Autodesk Inventor part; units mm, degrees
ref_plane "YZ Plane" through (0, 0, 0) normal (1, 0, 0) x (0, 1, 0)
ref_plane "XZ Plane" through (0, 0, 0) normal (0, 1, 0) x (-1, 0, 0)
ref_plane "XY Plane" through (0, 0, 0) normal (0, 0, 1) x (1, 0, 0)
sketch "Boceto1" plane through (0, 0, 0) normal (0, 1, 0) x (-1, 0, 0)
  circle A0 centre (0, 0) radius 7.95
  dimension "d0" = 15.9
extrude "Extrusión1" add sketch "Boceto1" along normal blind 1.3
sketch "Boceto2" plane through (0, 1.3, 0) normal (0, 1, 0) x (1, 0, 0)
  circle A0 centre (0, 0) radius 4.55
  dimension "d3" = 9.1
extrude "Extrusión2" add sketch "Boceto2" along normal blind 3.3
sketch "Boceto3" plane through (0, 4.6, 0) normal (0, 1, 0) x (1, 0, 0)
  circle A0 centre (0, 0) radius 3.05
  dimension "d6" = 6.1
extrude "Extrusión3" cut sketch "Boceto3" against normal blind 3.2
sketch "Boceto4" plane through (0, 1.4, 0) normal (0, 1, 0) x (1, 0, 0)
  arc A0 (0, -1.5) -> (0, 1.5) centre (0, 0) ccw
  line L0 (0, -1.5) -> (-7.8072, -1.5)
  circle A1 centre (0, 0) radius 7.95
  line L1 (0, 1.5) -> (-7.8072, 1.5)
  arc A2 (-7.8072, 1.5) -> (-7.8072, -1.5) centre (0, 0) ccw
  dimension "d9" = 3
extrude "Extrusión4" cut sketch "Boceto4" along normal blind 3.2 and the other way blind 1.6 contours L0 A1 L1 A0 picked at (-2.6447, -0.1676)
fillet "Empalme1" radius 0.3 1 edges at (4.55, 1.3, 0)
sketch "Boceto5" plane through (0, 0, 0) normal (0, -1, 0) x (1, 0, 0)
  arc A0 (-6.4786, -1.5) -> (-6.4786, 1.5) centre (0, 0) ccw
  arc A1 (-5.5509, -1.5) -> (-5.5509, 1.5) centre (0, 0) ccw
  line L0 (-7.8072, 1.5) -> (0, 1.5)
  line L1 (-5.5509, 1.5) -> (-6.4786, 1.5)
  line L2 (-7.8072, -1.5) -> (-4.6122, -1.5)
  line L3 (-6.4786, -1.5) -> (-5.5509, -1.5)
  dimension "d15" = 13.3
  dimension "d16" = 11.5
extrude "Extrusión5" add sketch "Boceto5" along normal blind 4.3
properties part number "Pieza_Presion_resorte" material "Plástico ABS"
Input: part model. Units: mm. Frame: model coordinates. A direction names the side the tool comes from. Give positions to 0.01 mm unless a question says otherwise; leave off trailing zeros. Write each loop counter-clockwise with the first axis right and the second up, starting at its lowest first coordinate (ties: lowest second). Pieces come first, ordered by that corner, then holes.
Q1. Section B-B, the plane z = 0. Output: boundary loops of the cut face in (x, y).
Q2. Section C-C, the plane y = -0.25. Output: boundary loops of the cut face in (x, z), plus the area to 3 significant figures.
Q3. Section D-D, the plane z = -6. Output: boundary loops of the cut face in (x, y), plus the area to 3 significant figures.
Q4. Material intervals for probe 1 along Z at (x, y) = (0, -3.15); probe 2 along Z at (x, y) = (0, 3.15); probe 3 along Y at (x, z) = (2.75, 0.5), sorted ascending.
Q5. First-contact query: P1, Ø8, axis at x = 1.5, z = -1.5, coming from the +Y side; P2, Ø4, axis at x = 2, y = 3, coming from the -Z side; P3, Ø4, axis at x = 6, z = 3, coming from the +Y side; P4, Ø8, axis at x = 0, z = 0, coming from the -Y side. Flat tips, straight axial feed; report the tip coordinate or a pass-through.
Q6. Set-up query: faces 1 (the face through (3.05, 3.02, 0.11)), 2 (the face through (-5, 1, -1.5)), 3 (the face through (5.745, -2.12, 0.232)), 4 (the face through (1, 4.6, -3.1)). Return all of +Z, -Z, +X, -X, +Y, -Y with unobstructed straight access to the full face (end or side cutting, diameter ignored); none if empty.
Q7. Pull-direction query (Z, two-part tool) for faces 5 (the face through (4.546, 3.079, -0.179)), 6 (the face through (1.5, 0.7, 0)), 7 (the face through (4, 1.3, -3)); classes: pulls with the +Z half, pulls with the -Z half, needs draft (parallel to the pull), parting line crosses it, or undercut.
Q8. Section A-A, the plane x = -6.25. Output: boundary loops of the cut face in (y, z).
Filled in:
1. outline: (1.5, 0) - (5.75, 0) - (5.75, -4.3) - (6.65, -4.3) - (6.65, 0) - (7.95, 0) - (7.95, 1.3) - (4.85, 1.3) arc R0.3 cw to (4.55, 1.6) - (4.55, 4.6) - (3.05, 4.6) - (3.05, 1.4) - (1.5, 1.4) - close
2. outline: (-6.48, -1.5) arc R6.65 ccw (long way) to (-6.48, 1.5) - (-5.55, 1.5) arc R5.75 cw (long way) to (-5.55, -1.5) - close
2. area: 32.3 mm2
3. outline: (-5.22, 0) - (-2.87, 0) - (-2.87, -4.3) - (2.87, -4.3) - (2.87, 0) - (5.22, 0) - (5.22, 1.3) - (-5.22, 1.3) - close
3. area: 38.2 mm2
4. probe 1: z = -6.65 to -5.75, 5.75 to 6.65
4. probe 2: z = -4.55 to -3.05, 3.05 to 4.55
4. probe 3: y = 0 to 1.4
5. P1: stops at y = 4.6
5. P2: stops at z = -7.89
5. P3: stops at y = 1.34
5. P4: stops at y = 0
6. face 1: +Y
6. face 2: -X, +Y, -Y
6. face 3: -Y
6. face 4: +Z, -Z, +X, -X, +Y
7. face 5: parting line crosses it
7. face 6: undercut
7. face 7: needs draft
8. outline: (-4.3, -2.27) - (0, -2.27) - (0, -4.91) - (1.3, -4.91) - (1.3, -1.5) - (-4.3, -1.5) - close; (-4.3, 1.5) - (1.3, 1.5) - (1.3, 4.91) - (0, 4.91) - (0, 2.27) - (-4.3, 2.27) - close
